Geometry: final body of the model. Coordinates: model frame, mm. Coordinates: 2 decimals unless noted, no trailing zeros. Write each loop counter-clockwise with the first axis right and the second up, starting at its lowest first coordinate (ties: lowest second). Pieces come first, ordered by that corner, then holes. Notation, with made-up numbers: (-29.5, 60.25) -> (6.5, 60.25) arc R17 ccw to (6.5, 73.25) -> close; hole circle Ø2 at (5.5, -38). An arc over 180 degrees is marked (long way). Answer as a JSON object with one key per item and string values. Group by question number.
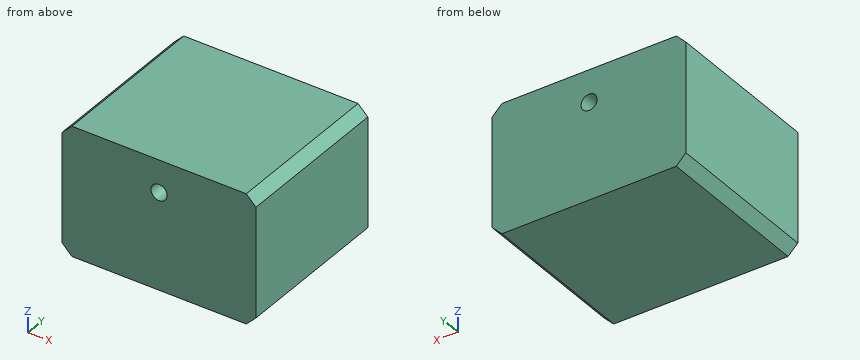
```python
from build123d import *

# Parameters (mm, degrees)
SKETCH_1_W          = 30
SKETCH_1_H          = 20
EXTRUDE_1_DEPTH     = 25
SKETCH_2_R          = 1.25
CUT_EXTRUDE_1_DEPTH = 31.822070015
CHAMFER_1_SIZE      = 1.5


with BuildPart() as part:
    # 草图1 → 凸台-拉伸1 (new body)
    with BuildSketch(Plane(origin=(0, 0, 0), x_dir=(1, 0, 0), z_dir=(0, 1, 0))):
        Rectangle(SKETCH_1_W, SKETCH_1_H)
    extrude(amount=EXTRUDE_1_DEPTH)

    # 草图2 → 切除-拉伸1 (cut, through all)
    with BuildSketch(Plane(origin=(0, 25, 0), x_dir=(1, 0, 0), z_dir=(0, 1, 0))):
        with Locations(Location((0, -5, 0), (0, 0, 270))):
            Circle(SKETCH_2_R)
    extrude(amount=-CUT_EXTRUDE_1_DEPTH, mode=Mode.SUBTRACT)

    # 倒角1
    chamfer_1_edges = [part.edges().sort_by_distance(p)[0] for p in [
        (-15, 12.5, -10),
        (15, 12.5, -10),
        (15, 12.5, 10),
        (-15, 12.5, 10),
    ]]
    chamfer(chamfer_1_edges, length=CHAMFER_1_SIZE)


solid = part.part
```
Item 1: Ray query, L1, parallel to X at y = 6, z = 5; L2, parallel to X at y = 9.5, z = 6. Return the intervals inside material, ascending. Write a range as [from, to].
Item 2: Section A-A on z = 5. Output: boundary loops of the cut face in (x, y), then the cut area to 4 significant figures.
Item 3: Section B-B on x = 0. Output: boundary loops of the cut face in (y, z), then the cut area to 4 significant figures.
Item 4: Section C-C on y = 6.75. Output: boundary loops of the cut face in (x, z).
Answer sheet:
{
 "1": {"L1": "x = [-15, -1.25], [1.25, 15]", "L2": "x = [-15, -0.75], [0.75, 15]"},
 "2": {"outline": "(-15, 0) -> (-1.25, 0) -> (-1.25, 25) -> (-15, 25) -> close; (1.25, 0) -> (15, 0) -> (15, 25) -> (1.25, 25) -> close", "area": "687.5 mm^2"},
 "3": {"outline": "(0, -10) -> (25, -10) -> (25, 3.75) -> (0, 3.75) -> close; (0, 6.25) -> (25, 6.25) -> (25, 10) -> (0, 10) -> close", "area": "437.5 mm^2"},
 "4": {"outline": "(-15, -8.5) -> (-13.5, -10) -> (13.5, -10) -> (15, -8.5) -> (15, 8.5) -> (13.5, 10) -> (-13.5, 10) -> (-15, 8.5) -> close; hole circle Ø2.5 at (0, 5)"}
}
